```python
from build123d import *

# Parameters (mm, degrees)
EXTRUDE_1_REACH              = 13.035
PATTERN_CIRCULAR_1_COUNT     = 12
CHAMFER_1_SIZE               = 0.2
HOLE_WIZARD_M3_1_D           = 3.2
HOLE_WIZARD_M3_1_DEPTH       = 10
HOLE_WIZARD_M3_1_CSINK_D     = 6.3
HOLE_WIZARD_M3_1_CSINK_ANGLE = 90
HOLE_WIZARD_M3_1_TIP         = 0.96137699


with BuildPart() as part:
    # 草图1 → 旋转1 (revolve)
    with BuildSketch(Plane.XY, mode=Mode.PRIVATE) as revolve_1_sk:
        Polygon((0, 2), (4.2, 2), (4.2, 5.2), (6.2, 5.2), (6.2, -1.5), (2, -1.5), (2, 0), (0, 0), align=None)
    revolve(revolve_1_sk.sketch.rotate(Axis((0, 0, 0), (0, -1, 0)), 90), axis=Axis((0, 0, 0), (0, -1, 0)))

    # 草图6 → 凸台-拉伸1 (add, up to next)
    with BuildSketch(Plane(origin=(0, 5.2, 0), x_dir=(1, 0, 0), z_dir=(0, 1, 0)), mode=Mode.PRIVATE) as extrude_1_sk1:
        with BuildLine():
            Line((-0.3, 4.189272013), (-0.15, 3.8))
            Line((-0.15, 3.8), (0.15, 3.8))
            Line((0.15, 3.8), (0.3, 4.189272013))
            ThreePointArc((0.3, 4.189272013), (0, 4.2), (-0.3, 4.189272013))
        make_face()
    extrude_1_tool1 = extrude(extrude_1_sk1.sketch, amount=-EXTRUDE_1_REACH, mode=Mode.PRIVATE) - part.part
    extrude_1 = extrude_1_tool1.solids().sort_by_distance((0, 5.2, -4.020503))[0]
    add(extrude_1)

    # 阵列(圆周)1: 凸台-拉伸1 ×12 about axis
    pattern_circular_1_axis = Axis((0, 0, 0.0130623), (0, 1, 0))
    for i in range(1, PATTERN_CIRCULAR_1_COUNT):
        add(extrude_1.rotate(pattern_circular_1_axis, i * 360 / PATTERN_CIRCULAR_1_COUNT))

    # 倒角1
    chamfer_1_edges = [part.edges().sort_by_distance(p)[0] for p in [
        (-0.220099646, 5.2, 4.008043467),
        (0.220099646, 5.2, 4.008043467),
        (0, 5.2, 3.8261246),
        (2.963047356, 5.2, 2.976634066),
        (1.806983311, 5.2, 3.583533316),
        (2.188995086, 5.2, 3.363488592),
        (1.90653115, 5.2, 3.315271118),
        (4.053472149, 5.2, 1.099710659),
        (3.351583041, 5.2, 2.2034896),
        (3.573571791, 5.2, 1.820532654),
        (3.302208818, 5.2, 1.91959345),
        (4.060265001, 5.2, -1.0743594),
        (4.000883833, 5.2, 0.235436447),
        (4.001779561, 5.2, -0.209657003),
        (3.8130623, 5.2, 0.0130623),
        (2.976633055, 5.2, -2.963048372),
        (3.579482315, 5.2, -1.795336429),
        (3.356386981, 5.2, -2.183312937),
        (3.302208818, 5.2, -1.89346885),
        (1.090435686, 5.2, -4.055977073),
        (2.197803646, 5.2, -3.344478358),
        (1.808889205, 5.2, -3.569542645),
        (1.90653115, 5.2, -3.289146518),
        (-1.090435686, 5.2, -4.055977073),
        (-0.225, 5.2, -3.994636007),
        (0, 5.2, -3.8),
        (0.225, 5.2, -3.994636007),
        (-2.976633055, 5.2, -2.963048372),
        (-1.808889205, 5.2, -3.569542645),
        (-2.197803646, 5.2, -3.344478358),
        (-1.90653115, 5.2, -3.289146518),
        (-4.060265001, 5.2, -1.0743594),
        (-3.356386981, 5.2, -2.183312937),
        (-3.579482315, 5.2, -1.795336429),
        (-3.302208818, 5.2, -1.89346885),
        (-4.053472149, 5.2, 1.099710659),
        (-4.001779561, 5.2, -0.209657003),
        (-4.000883833, 5.2, 0.235436447),
        (-3.8130623, 5.2, 0.0130623),
        (-2.963047356, 5.2, 2.976634066),
        (-3.573571791, 5.2, 1.820532654),
        (-3.351583041, 5.2, 2.2034896),
        (-3.302208818, 5.2, 1.91959345),
        (0, 5.2, -6.2),
        (-1.083642839, 5.2, 4.05779721),
        (-2.188995086, 5.2, 3.363488592),
        (-1.806983311, 5.2, 3.583533316),
        (-1.90653115, 5.2, 3.315271118),
        (1.083642839, 5.2, 4.05779721),
    ]]
    chamfer(chamfer_1_edges, length=CHAMFER_1_SIZE)

    # M3 平头机械螺钉的锥形沉头孔1
    with Locations(Plane(origin=(0, 2, 0), x_dir=(1, 0, 0), z_dir=(0, 1, 0))):
        with Locations((0, 0)):
            CounterSinkHole(HOLE_WIZARD_M3_1_D / 2, HOLE_WIZARD_M3_1_CSINK_D / 2, depth=HOLE_WIZARD_M3_1_DEPTH, counter_sink_angle=HOLE_WIZARD_M3_1_CSINK_ANGLE)
            with Locations((0, 0, -(HOLE_WIZARD_M3_1_DEPTH + HOLE_WIZARD_M3_1_TIP / 2))):  # 118° drill point
                Cone(0, HOLE_WIZARD_M3_1_D / 2, HOLE_WIZARD_M3_1_TIP, mode=Mode.SUBTRACT)


solid = part.part
```
For this review, take the finished solid that the model builds, in its own axes (mm). A direction names the side the tool comes from. Coordinates: 2 decimals unless noted, no trailing zeros. Write each loop counter-clockwise with the first axis right and the second up, starting at its lowest first coordinate (ties: lowest second). Pieces come first, ordered by that corner, then holes. Notation, with made-up numbers: (65.5, 85.5) - (111.5, 85.5) arc R28 cw to (111.5, 123.5) - close; hole circle Ø5 at (34, 82). An arc over 180 degrees is marked (long way). Answer in a Markdown table with one row per item. Add a question column.
Q1. Draft analysis for pull direction X (two halves, no side actions). For faces 4 (the cylindrical face through (2.97, 3.52, -2.97)), 5 (the flat face through (0, -1.5, 3)), 6 (the cylindrical face through (-1.9, 1.7, 5.9)), state which applies: +X half, -X half, draft (parallel to the pull), parting line (faces both ways), or undercut.
Q2. For P1, Ø2, axis at x = 5, y = 4, coming from the +Z side; P2, Ø1, axis at x = -2, y = 1.5, coming from the -Z side; P3, Ø2.5, axis at x = 0, z = 0, coming from the +Y side; P4, Ø2.5, axis at x = -1, z = -0.5, coming from the +Y side, all flat-tipped, find the tip position at first contact; note any pin that passes through.
Q3. We need section A-A, the plane y = -0.25. State the section outline as (x, z) points.
Q4. Tool access review of faces 1 (the cylindrical face through (-2.96, 3.52, 2.98)), 2 (the cylindrical face through (2, -1, 0)), 3 (the flat face through (-4, 5.2, 3)): name each direction out of +Z, -Z, +X, -X, +Y, -Y from which nothing blocks a thin tool from reaching the whole face with its end or side.
Q5. For probe 1 along X at (y, z) = (-0.95, 0); probe 2 along X at (y, z) = (4.5, 3); probe 3 along Z at (x, y) = (-1.5, 3.25), list the stretches that pass through material, from the lowest coordinate up.
Answer list:
| question | item | result |
|---|---|---|
| 1 | face 4 | undercut |
| 1 | face 5 | draft |
| 1 | face 6 | parting line |
| 2 | P1 | stops at z = 4.74 |
| 2 | P2 | stops at z = -6.02 |
| 2 | P3 | passes through |
| 2 | P4 | stops at y = 1.22 |
| 3 | outline | circle Ø12.4 at (0, 0); hole circle Ø4 at (0, 0) |
| 4 | face 1 | +Y |
| 4 | face 2 | -Y |
| 4 | face 3 | +Z, -Z, +X, -X, +Y |
| 5 | probe 1 | x = -6.2 to -2, 2 to 6.2 |
| 5 | probe 2 | x = -5.43 to -2.94, 2.94 to 5.43 |
| 5 | probe 3 | z = -6.02 to -3.92, 3.92 to 6.02 |
